Verification items for the finished model (mm, model axes). A direction names the side the tool comes from. Round coordinates to 2 decimals unless told otherwise and drop trailing zeros. Write each loop counter-clockwise with the first axis right and the second up, starting at its lowest first coordinate (ties: lowest second). Pieces come first, ordered by that corner, then holes. Notation, with made-up numbers: M 88.25,43 L 110.25,43 A19 ccw 110.25,73 Z; hole C 25.5,81.5 d10. An arc over 180 degrees is marked long. One line per question, with ' | ' between items.
from build123d import *

# Parameters (mm, degrees)
RESSALTO_EXTRUS_O1_DEPTH        = 5
FURO_ROSCADO_DE_M82_D           = 6.8
FURO_ROSCADO_DE_M82_CSINK_D     = 8.05
FURO_ROSCADO_DE_M82_CSINK_ANGLE = 90


with BuildPart() as part:
    # Esboço1 → Ressalto-extrusão1 (new, symmetric)
    with BuildSketch(Plane(origin=(0, 0, 0), x_dir=(1, 0, 0), z_dir=(0, 1, 0))):
        Polygon((70, 24), (150, 24), (150, 50), (-150, 50), (-150, -50), (150, -50), (150, -24), (70, -24), align=None)
    extrude(amount=RESSALTO_EXTRUS_O1_DEPTH, both=True)

    # Furo roscado de M82 (through all)
    with Locations(Plane(origin=(-135, 5, -17), x_dir=(0, 0, 1), z_dir=(0, 1, 0))):
        with Locations((0, 0), (34, 0), (34, 60), (0, 60)):
            CounterSinkHole(FURO_ROSCADO_DE_M82_D / 2, FURO_ROSCADO_DE_M82_CSINK_D / 2, counter_sink_angle=FURO_ROSCADO_DE_M82_CSINK_ANGLE)


solid = part.part
1. Mould release check, pull along Z, two halves, no side actions. Record for faces 3 (the face through (-2, -5, -1)), 4 (the face through (70, 0, 0)), 5 (the face through (2, 0, -50)): pulls with the +Z half, pulls with the -Z half, needs draft (parallel to the pull), parting line crosses it, or undercut.
Results:
face 3: needs draft | face 4: undercut | face 5: pulls with the -Z half
2. Tool access check on faces 1 (the face through (-2, 5, -1)), 2 (the face through (111, 0, 24)). Record the directions out of +Z, -Z, +X, -X, +Y, -Y that give a thin tool (end or side, any length) a straight path to the whole face; none if there is none.
Results:
face 1: +Z, -Z, +X, -X, +Y | face 2: +X, +Y, -Y
3. Section check A-A, the plane z = 17. Record the cut outline in (x, y) (3 decimals).
Results:
outline: M -150,-5 L -138.4,-5 L -138.4,4.375 L -139.025,5 L -150,5 Z; M -131.6,-5 L -78.4,-5 L -78.4,4.375 L -79.025,5 L -130.975,5 L -131.6,4.375 Z; M -71.6,-5 L 70,-5 L 70,5 L -70.975,5 L -71.6,4.375 Z
4. Thickness scan on line 1 (Z direction, x = -135, y = -2.25); line 2 (X direction, y = 1.25, z = 17); line 3 (Z direction, x = 75, y = -0.75). Record the ranges inside material, lowest first.
Results:
line 1: z = -50 to -20.4, -13.6 to 13.6, 20.4 to 50 | line 2: x = -150 to -138.4, -131.6 to -78.4, -71.6 to 70 | line 3: z = -50 to -24, 24 to 50
5. Section check B-B, the plane x = -75. Record the cut outline in (y, z) (3 decimals), then the cut area to 3 significant figures.
Results:
outline: M -5,-50 L 5,-50 L 5,-21.025 L 4.375,-20.4 L -5,-20.4 Z; M -5,-13.6 L 4.375,-13.6 L 5,-12.975 L 5,12.975 L 4.375,13.6 L -5,13.6 Z; M -5,20.4 L 4.375,20.4 L 5,21.025 L 5,50 L -5,50 Z | area: 863 mm2
6. Go/stop test with flat-tipped pins: P1, Ø5.5, axis at x = -135, z = -17, coming from the +Y side; P2, Ø9, axis at x = -75, z = 17, coming from the -Y side. Record where each tip stops, or that it passes through.
Results:
P1: passes through | P2: stops at y = -5
7. Section check C-C, the plane y = -1.5. Record the cut outline in (x, z).
Results:
outline: M -150,-50 L 150,-50 L 150,-24 L 70,-24 L 70,24 L 150,24 L 150,50 L -150,50 Z; hole C -135,-17 d6.8; hole C -135,17 d6.8; hole C -75,-17 d6.8; hole C -75,17 d6.8
8. Section check D-D, the plane x = 83.5. Record the cut outline in (y, z), then the cut area to 3 significant figures.
Results:
outline: M -5,-50 L 5,-50 L 5,-24 L -5,-24 Z; M -5,24 L 5,24 L 5,50 L -5,50 Z | area: 520 mm2
